```python
from build123d import *
from OCP.BRepFilletAPI import BRepFilletAPI_MakeChamfer

# Parameters (mm, degrees)
CROQUIS1_W              = 105
CROQUIS1_H              = 150
SALIENTE_EXTRUIR1_DEPTH = 8
CROQUIS2_R              = 1.3
CROQUIS2_R_2            = 1.5
CORTAR_EXTRUIR4_DEPTH   = 8
CROQUIS3_W              = 52.4
CROQUIS3_H              = 27
SALIENTE_EXTRUIR2_DEPTH = 6
REDONDEO1_R             = 8
REDONDEO2_R             = 8
REDONDEO3_R             = 8
REDONDEO4_R             = 8
CORTAR_EXTRUIR5_DEPTH   = 2
CHAFL_N1_SIZE           = 2
CHAFL_N1_SIZE2          = 1.154700538
CHAFL_N2_SIZE           = 2
CHAFL_N2_SIZE2          = 3.464101615
CORTAR_EXTRUIR6_DEPTH   = 8
CORTAR_EXTRUIR7_DEPTH   = 2.45
CHAFL_N3_SIZE           = 0.5
CHAFL_N3_SIZE2          = 0.866025404
CROQUIS9_R              = 1.3
CORTAR_EXTRUIR9_DEPTH   = 8


with BuildPart() as part:
    # Croquis1 → Saliente-Extruir1 (new body)
    with BuildSketch(Plane.XY):
        with Locations((52.5, 75)):
            Rectangle(CROQUIS1_W, CROQUIS1_H)
    extrude(amount=SALIENTE_EXTRUIR1_DEPTH)

    # Croquis2 → Cortar-Extruir4 (cut)
    with BuildSketch(Plane.XY.offset(8)):
        with Locations((52.5, 137)):
            Circle(CROQUIS2_R)
        with Locations((47.5, 142)):
            Circle(CROQUIS2_R_2)
        with Locations((47.5, 132)):
            Circle(CROQUIS2_R_2)
        with Locations(Location((57.5, 132, 0), (0, 0, 180))):
            Circle(CROQUIS2_R_2)
        with Locations(Location((57.5, 142, 0), (0, 0, 180))):
            Circle(CROQUIS2_R_2)
        with BuildLine():
            Line((19.25, 108), (19.25, 15))
            ThreePointArc((19.25, 15), (15, 10.75), (10.75, 15))
            Line((10.75, 15), (10.75, 108))
            ThreePointArc((10.75, 108), (15, 112.25), (19.25, 108))
        make_face()
        with BuildLine():
            Line((85.75, 108), (85.75, 15))
            ThreePointArc((85.75, 15), (90, 10.75), (94.25, 15))
            Line((94.25, 15), (94.25, 108))
            ThreePointArc((94.25, 108), (90, 112.25), (85.75, 108))
        make_face()
    extrude(amount=-CORTAR_EXTRUIR4_DEPTH, mode=Mode.SUBTRACT)

    # Croquis3 → Saliente-Extruir2 (add)
    with BuildSketch(Plane.XY.offset(8)):
        with Locations((52.5, 136.5)):
            Rectangle(CROQUIS3_W, CROQUIS3_H)
        Polygon((74.7, 127), (52.5, 127), (30.3, 127), (30.3, 147.1), (74.7, 147.1), align=None, mode=Mode.SUBTRACT)
    extrude(amount=SALIENTE_EXTRUIR2_DEPTH)

    # Redondeo1
    redondeo1_edges = [part.edges().sort_by_distance(p)[0] for p in [
        (0, 150, 4),
    ]]
    fillet(redondeo1_edges, radius=REDONDEO1_R)

    # Redondeo2
    redondeo2_edges = [part.edges().sort_by_distance(p)[0] for p in [
        (105, 150, 4),
    ]]
    fillet(redondeo2_edges, radius=REDONDEO2_R)

    # Redondeo3
    redondeo3_edges = [part.edges().sort_by_distance(p)[0] for p in [
        (0, 0, 4),
    ]]
    fillet(redondeo3_edges, radius=REDONDEO3_R)

    # Redondeo4
    redondeo4_edges = [part.edges().sort_by_distance(p)[0] for p in [
        (105, 0, 4),
    ]]
    fillet(redondeo4_edges, radius=REDONDEO4_R)

    # Croquis4 → Cortar-Extruir5 (cut)
    # profile 1 of 2: a face of its own
    with BuildSketch(Plane.XY.offset(8)):
        with BuildLine():
            Line((27, 108), (27, 15))
            ThreePointArc((27, 15), (15, 3), (3, 15))
            Line((3, 15), (3, 108))
            ThreePointArc((3, 108), (15, 120), (27, 108))
        make_face()
        with BuildLine():
            Line((10.75, 108), (10.75, 15))
            ThreePointArc((10.75, 15), (15, 10.75), (19.25, 15))
            Line((19.25, 15), (19.25, 108))
            ThreePointArc((19.25, 108), (15, 112.25), (10.75, 108))
        make_face(mode=Mode.SUBTRACT)
    # profile 2 of 2: a face of its own
    with BuildSketch(Plane.XY.offset(8)):
        with BuildLine():
            Line((78, 108), (78, 15))
            ThreePointArc((78, 15), (90, 3), (102, 15))
            Line((102, 15), (102, 108))
            ThreePointArc((102, 108), (90, 120), (78, 108))
        make_face()
        with BuildLine():
            Line((85.75, 108), (85.75, 15))
            ThreePointArc((85.75, 15), (90, 10.75), (94.25, 15))
            Line((94.25, 15), (94.25, 108))
            ThreePointArc((94.25, 108), (90, 112.25), (85.75, 108))
        make_face(mode=Mode.SUBTRACT)
    extrude(amount=-CORTAR_EXTRUIR5_DEPTH, mode=Mode.SUBTRACT)

    # Chaflán1: one chamfer whose edges measure the first distance from different faces: ONE call of the kernel's chamfer builder (chamfer() names one face for all edges)
    chafl_n1_edges_1 = [part.edges().sort_by_distance(p)[0] for p in [
        (52.5, 127, 14),
    ]]
    chafl_n1_side_1 = [part.faces().sort_by_distance(p)[0] for p in [
        (52.5, 127, 11),
    ]]
    chafl_n1_edges_2 = [part.edges().sort_by_distance(p)[0] for p in [
        (30.3, 137.05, 14),
    ]]
    chafl_n1_side_2 = [part.faces().sort_by_distance(p)[0] for p in [
        (30.3, 137.05, 11),
    ]]
    chafl_n1_edges_3 = [part.edges().sort_by_distance(p)[0] for p in [
        (52.5, 147.1, 14),
    ]]
    chafl_n1_side_3 = [part.faces().sort_by_distance(p)[0] for p in [
        (52.5, 147.1, 11),
    ]]
    chafl_n1_edges_4 = [part.edges().sort_by_distance(p)[0] for p in [
        (74.7, 137.05, 14),
    ]]
    chafl_n1_side_4 = [part.faces().sort_by_distance(p)[0] for p in [
        (74.7, 137.05, 11),
    ]]
    chafl_n1 = BRepFilletAPI_MakeChamfer(part.part.solid().wrapped)
    for e in chafl_n1_edges_1:
        chafl_n1.Add(CHAFL_N1_SIZE, CHAFL_N1_SIZE2, e.wrapped, chafl_n1_side_1[0].wrapped)  # the first distance lies on this face
    for e in chafl_n1_edges_2:
        chafl_n1.Add(CHAFL_N1_SIZE, CHAFL_N1_SIZE2, e.wrapped, chafl_n1_side_2[0].wrapped)  # the first distance lies on this face
    for e in chafl_n1_edges_3:
        chafl_n1.Add(CHAFL_N1_SIZE, CHAFL_N1_SIZE2, e.wrapped, chafl_n1_side_3[0].wrapped)  # the first distance lies on this face
    for e in chafl_n1_edges_4:
        chafl_n1.Add(CHAFL_N1_SIZE, CHAFL_N1_SIZE2, e.wrapped, chafl_n1_side_4[0].wrapped)  # the first distance lies on this face
    add(Compound.cast(chafl_n1.Shape()), mode=Mode.REPLACE)

    # Chaflán2
    chafl_n2_edges = [part.edges().sort_by_distance(p)[0] for p in [
        (52.5, 123, 8),
        (78.7, 136.5, 8),
        (26.3, 136.5, 8),
    ]]
    chafl_n2_side = [part.faces().sort_by_distance(p)[0] for p in [
        (52.5, 73.36933007, 8),
    ]]
    chamfer(chafl_n2_edges, length=CHAFL_N2_SIZE, length2=CHAFL_N2_SIZE2, reference=chafl_n2_side[0])

    # Croquis6 → Cortar-Extruir6 (cut)
    with BuildSketch(Plane.XY.offset(8)):
        with BuildLine():
            Line((37, 20), (68, 20))
            ThreePointArc((68, 20), (70.5, 17.5), (68, 15))
            Line((68, 15), (37, 15))
            ThreePointArc((37, 15), (34.5, 17.5), (37, 20))
        make_face()
        with BuildLine():
            Line((37, 30), (68, 30))
            ThreePointArc((68, 30), (70.5, 32.5), (68, 35))
            Line((68, 35), (37, 35))
            ThreePointArc((37, 35), (34.5, 32.5), (37, 30))
        make_face()
        with BuildLine():
            Line((37, 45), (68, 45))
            ThreePointArc((68, 45), (70.5, 47.5), (68, 50))
            Line((68, 50), (37, 50))
            ThreePointArc((37, 50), (34.5, 47.5), (37, 45))
        make_face()
        with BuildLine():
            Line((37, 60), (68, 60))
            ThreePointArc((68, 60), (70.5, 62.5), (68, 65))
            Line((68, 65), (37, 65))
            ThreePointArc((37, 65), (34.5, 62.5), (37, 60))
        make_face()
        with BuildLine():
            Line((37, 75), (68, 75))
            ThreePointArc((68, 75), (70.5, 77.5), (68, 80))
            Line((68, 80), (37, 80))
            ThreePointArc((37, 80), (34.5, 77.5), (37, 75))
        make_face()
        with BuildLine():
            Line((37, 90), (68, 90))
            ThreePointArc((68, 90), (70.5, 92.5), (68, 95))
            Line((68, 95), (37, 95))
            ThreePointArc((37, 95), (34.5, 92.5), (37, 90))
        make_face()
        with BuildLine():
            Line((37, 105), (68, 105))
            ThreePointArc((68, 105), (70.5, 107.5), (68, 110))
            Line((68, 110), (37, 110))
            ThreePointArc((37, 110), (34.5, 107.5), (37, 105))
        make_face()
    extrude(amount=-CORTAR_EXTRUIR6_DEPTH, mode=Mode.SUBTRACT)

    # Croquis8 → Cortar-Extruir7 (cut)
    with BuildSketch(Plane(origin=(0, 0, 0), x_dir=(-1, 0, 0), z_dir=(0, 0, -1))):
        Polygon((-52.5, 140.175426481), (-55.25, 138.58771324), (-55.25, 135.41228676), (-52.5, 133.824573519), (-49.75, 135.41228676), (-49.75, 138.58771324), align=None)
        Polygon((-64.7, 140.202903958), (-67.45, 138.615190718), (-67.45, 135.439764237), (-64.7, 133.852050997), (-61.95, 135.439764237), (-61.95, 138.615190718), align=None)
        Polygon((-37.55, 138.615190718), (-40.3, 140.202903958), (-43.05, 138.615190718), (-43.05, 135.439764237), (-40.3, 133.852050997), (-37.55, 135.439764237), align=None)
    extrude(amount=-CORTAR_EXTRUIR7_DEPTH, mode=Mode.SUBTRACT)

    # Chaflán3
    chafl_n3_edges = [part.edges().sort_by_distance(p)[0] for p in [
        (66.075, 134.645907617, 0),
        (63.325, 134.645907617, 0),
        (61.95, 137.027477477, 0),
        (63.325, 139.409047338, 0),
        (66.075, 139.409047338, 0),
        (67.45, 137.027477477, 0),
        (41.675, 139.409047338, 0),
        (43.05, 137.027477477, 0),
        (41.675, 134.645907617, 0),
        (38.925, 134.645907617, 0),
        (37.55, 137.027477477, 0),
        (38.925, 139.409047338, 0),
        (49.75, 137, 0),
        (51.125, 139.38156986, 0),
        (53.875, 139.38156986, 0),
        (55.25, 137, 0),
        (53.875, 134.61843014, 0),
        (51.125, 134.61843014, 0),
    ]]
    chafl_n3_side = [part.faces().sort_by_distance(p)[0] for p in [
        (52.5, 1.830983342, 0),
    ]]
    chamfer(chafl_n3_edges, length=CHAFL_N3_SIZE, length2=CHAFL_N3_SIZE2, reference=chafl_n3_side[0])

    # Croquis9 → Cortar-Extruir9 (cut)
    with BuildSketch(Plane(origin=(0, 0, 0), x_dir=(-1, 0, 0), z_dir=(0, 0, -1))):
        with Locations((-64.7, 137.027477477)):
            Circle(CROQUIS9_R)
        with Locations((-40.3, 137.027477477)):
            Circle(CROQUIS9_R)
    extrude(amount=-CORTAR_EXTRUIR9_DEPTH, mode=Mode.SUBTRACT)


solid = part.part
```
Work out the finished part from the listing and answer in its coordinate system (mm). A direction names the side the tool comes from. Coordinates: 2 decimals unless noted, no trailing zeros. Loops run counter-clockwise (first coordinate to the right, second up) from the corner with the lowest first, then second, coordinate; pieces in that order, holes last. Notation, with made-up numbers: M -2,30 L 14,30 A22 ccw 14,44 Z; hole C 2.5,33 d9. An arc over 180 degrees is marked long. Use CSV: the item, a comma, the result in double quotes. Start each with the question number.
(1) For a pull along Y with two mould halves and no side action, classify faces 1 (the face through (52, 59, 8)), 2 (the face through (52, 150, 5)), 3 (the face through (39, 136, 2.45)), 4 (the face through (53, 80, 4)) as +Y half, -Y half, draft (parallel to the pull), parting line (faces both ways), or undercut.
(2) Find section C-C, the plane z = 9.5. Give the vertices of the cut face in (x, y), then the cut area to 3 significant figures.
(3) Find section A-A, the plane x = 90. Give the vertices of the cut face in (y, z).
(4) Consider line 1 (X direction, y = 100.5, z = 1.5); line 2 (X direction, y = 142, z = 4.25); line 3 (Z direction, x = 79, y = 85). Determine where each line is inside the solid, lowest interval first.
(5) For faces 5 (the face through (19.25, 62, 3)), 6 (the face through (25.314, 135.297, 9.756)), 7 (the face through (66, 136, 2.45)), 8 (the face through (15, 120, 7)), determine the directions among +Z, -Z, +X, -X, +Y, -Y from which every point of the face is accessible in a straight line to the end or side of a thin tool.
(6) Given pin 1 Ø5 at (x, y) = (47.5, 132) entering from +Z; pin 2 Ø1.8 at (x, y) = (47.5, 142) entering from -Z (3 decimals); pin 3 Ø1.5 at (x, z) = (41.5, 12) entering from -Y; pin 4 Ø1.3 at (y, z) = (141, 12) entering from -X, each flat-ended and moving along its own axis, determine where each tip first touches the part or whether it passes through.
(7) Find section B-B, the plane y = 77.5. Give the vertices of the cut face in (x, z), then the cut area to 3 significant figures.
Recorded:
1,face 1,"draft"
1,face 2,"+Y half"
1,face 3,"undercut"
1,face 4,"undercut"
2,outline,"M 25.17,121.87 L 79.83,121.87 L 79.83,150 L 25.17,150 Z; hole M 30.3,127 L 74.7,127 L 74.7,147.1 L 30.3,147.1 Z"
2,area,"646 mm^2"
3,outline,"M 0,0 L 10.75,0 L 10.75,6 L 3,6 L 3,8 L 0,8 Z; M 112.25,0 L 150,0 L 150,8 L 120,8 L 120,6 L 112.25,6 Z"
4,line 1,"x = 0 to 10.75, 19.25 to 85.75, 94.25 to 105"
4,line 2,"x = 0 to 46, 49 to 56, 59 to 105"
4,line 3,"z = 0 to 6"
5,face 5,"+Z, -Z"
5,face 6,"+Z, -X, +Y, -Y"
5,face 7,"-Z"
5,face 8,"+Z"
6,pin 1,"stops at z = 8"
6,pin 2,"passes through"
6,pin 3,"stops at y = 122.88"
6,pin 4,"stops at x = 26.23"
7,outline,"M 0,0 L 10.75,0 L 10.75,6 L 3,6 L 3,8 L 0,8 Z; M 19.25,0 L 34.5,0 L 34.5,8 L 27,8 L 27,6 L 19.25,6 Z; M 70.5,0 L 85.75,0 L 85.75,6 L 78,6 L 78,8 L 70.5,8 Z; M 94.25,0 L 105,0 L 105,8 L 102,8 L 102,6 L 94.25,6 Z"
7,area,"354 mm^2"
